Design review of the part built by this model. Coordinates are the model's own, in mm. Face numbers are marked on the shaded views. Coordinates: 2 decimals unless noted, no trailing zeros. Write each loop counter-clockwise with the first axis right and the second up, starting at its lowest first coordinate (ties: lowest second). Pieces come first, ordered by that corner, then holes. Notation, with made-up numbers: (-16, 78) -> (-4, 78) arc R19 cw to (-4, 97) -> close; hole circle Ø7 at (-35.5, -4). An arc over 180 degrees is marked (long way). Return JSON: item names as keys, results as strings. Group by question number.
Autodesk Inventor part; units mm, degrees
ref_plane "YZ Plane" through (0, 0, 0) normal (1, 0, 0) x (0, 1, 0)
ref_plane "XZ Plane" through (0, 0, 0) normal (0, 1, 0) x (-1, 0, 0)
ref_plane "XY Plane" through (0, 0, 0) normal (0, 0, 1) x (1, 0, 0)
sketch "Sketch1" plane through (0, 0, 0) normal (0, 1, 0) x (-1, 0, 0)
  line L0 (0, 0) -> (114.3, 0)
  line L1 (114.3, 0) -> (114.3, -88.9)
  line L2 (114.3, -88.9) -> (0, -88.9)
  line L3 (0, -88.9) -> (0, 0)
  line L4 (114.3, 0) -> (0, 0)
  line L5 (0, 0) -> (0, 6.35)
  line L6 (0, 6.35) -> (114.3, 6.35)
  line L7 (114.3, 6.35) -> (114.3, 0)
  line L8 (114.3, -88.9) -> (0, -88.9)
  line L9 (0, -88.9) -> (0, -95.25)
  line L10 (0, -95.25) -> (114.3, -95.25)
  line L11 (114.3, -95.25) -> (114.3, -88.9)
  dimension "d0" = 114.3
  dimension "d1" = 88.9
  dimension "d2" = 6.35
  dimension "d3" = 6.35
extrude "Extrusion1" add sketch "Sketch1" along normal blind 6.35 contours L0 L1 L2 L3
extrude "Extrusion2" add sketch "Sketch1" along normal blind 25.4 contours L5 L6 L7 L0 | L2 L11 L10 L9
properties part number "marker relese plate"
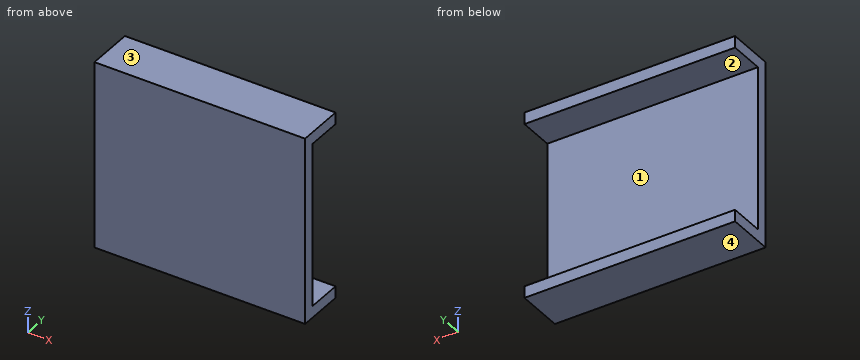
Q1. We need section B-B on x = -61. Write out the cut boundary in (y, z), plus the area to 3 significant figures.
Q2. For P1, Ø4, axis at x = -82.5, z = -17.5, coming from the +Y side, flat-tipped, find the tip position at first contact; note if it passes through.
Q3. We need section A-A on y = 18.5. Write out the cut boundary in (x, z), plus the area to 3 significant figures.
Q4. We need section C-C on z = -9. Write out the cut boundary in (x, y).
Q5. Wall thickness on L1, parallel to Z at x = -29.5, y = 13.5; L2, parallel to Y at x = -96, z = -28: over which ranges is each line inside the solid? List them lowest first.
Q6. The part is to be moulded in two halves that separate along Z. For the marked faces 1, 2, 3 and 4, say which applies: +Z half, -Z half, draft (parallel to the pull), parting line (faces both ways), or undercut.
Findings below:
{
 "1": {"outline": "(0, -95.25) -> (25.4, -95.25) -> (25.4, -88.9) -> (6.35, -88.9) -> (6.35, 0) -> (25.4, 0) -> (25.4, 6.35) -> (0, 6.35) -> close", "area": "887 mm^2"},
 "2": {"P1": "stops at y = 6.35"},
 "3": {"outline": "(-114.3, -95.25) -> (0, -95.25) -> (0, -88.9) -> (-114.3, -88.9) -> close; (-114.3, 0) -> (0, 0) -> (0, 6.35) -> (-114.3, 6.35) -> close", "area": "1,450 mm^2"},
 "4": {"outline": "(-114.3, 0) -> (0, 0) -> (0, 6.35) -> (-114.3, 6.35) -> close"},
 "5": {"L1": "z = -95.25 to -88.9, 0 to 6.35", "L2": "y = 0 to 6.35"},
 "6": {"face 1": "undercut", "face 2": "undercut", "face 3": "+Z half", "face 4": "-Z half"}
}
